Verification items for the finished model (mm, model axes). A direction names the side the tool comes from. Coordinates: 2 decimals unless noted, no trailing zeros. Order: outer loops, then holes, each group sorted by start corner. A loop starts at its lowest first (then second) coordinate and runs counter-clockwise, first axis right, second up.
Q1. Cross-section at C-C, the plane z = 8.5. Record the boundary of the cut face in (x, y).
Q2. Cross-section at D-D, the plane z = 2.5. Record the boundary of the cut face in (x, y).
Q3. Thickness scan on line 1 (Y direction, x = 20.5, z = 5.5); line 2 (Y direction, x = -38.5, z = 4.25); line 3 (X direction, y = -21, z = 4.5). Record the ranges inside material, lowest first.
Q4. Set-up check for faces 1 (the flat face through (15.98, 33.95, 2.53)), 2 (the flat face through (-28, 16, 10)), 3 (the cylindrical face through (16.71, 32.91, 8.5)): record each of +Z, -Z, +X, -X, +Y, -Y from which the full face is reachable in a straight line by a thin tool's end or side.
Q5. Depth check by flat-ended pin: P1, Ø3, axis at x = -38.5, z = 7, coming from the +Y side; P2, Ø1, axis at x = 11.5, z = 6.5, coming from the +Y side; P3, Ø3, axis at y = -21, z = 8, coming from the -X side. Enter the tip coordinate at first touch or a pass-through.
from build123d import *

# Parameters (mm, degrees)
F1_DEPTH = 10
F2_R     = 5
F3_SIZE  = 4.99999


# Not quite as in the source:
# - a fillet or chamfer is up to 0.001 mm smaller than in the source, because OpenCascade refuses the exact size


with BuildPart() as f1:
    # F0 (on Top) → F1 (new body)
    with BuildSketch(Plane.XY):
        Polygon((42.2499991953, 60.7764059144), (-57.7500008047, 60.7764059144), (-57.7500008047, -53.026408835), (-33.2429584743, -53.026408835), (-5.9190154745, 31.4806343348), (42.2499991953, 31.4806343348), align=None)
    extrude(amount=F1_DEPTH)

    # F2
    f2_edges = [f1.edges().sort_by_distance(p)[0] for p in [
        (-57.750001, 3.874999, 10),
        (-19.580987, -10.772887, 10),
        (-45.49648, -53.026409, 10),
        (18.165492, 31.480634, 10),
        (-7.750001, 60.776406, 10),
        (42.249999, 46.12852, 10),
    ]]
    fillet(f2_edges, radius=F2_R)

    # F3 (size 5 in the source; OpenCascade refuses exactly that, so slightly less here)
    f3_edges = [f1.edges().sort_by_distance(p)[0] for p in [
        (18.165492, 31.480634, 0),
        (42.249999, 46.12852, 0),
        (-7.750001, 60.776406, 0),
        (-57.750001, 3.874999, 0),
        (-45.49648, -53.026409, 0),
        (-19.580987, -10.772887, 0),
    ]]
    chamfer(f3_edges, length=F3_SIZE)


solid = f1.part
Check values:
1. outline: (-56.32, -51.6) - (-34.28, -51.6) - (-6.96, 32.91) - (40.82, 32.91) - (40.82, 59.35) - (-56.32, 59.35) - close
2. outline: (-55.25, -50.53) - (-35.06, -50.53) - (-7.74, 33.98) - (39.75, 33.98) - (39.75, 58.28) - (-55.25, 58.28) - close
3. line 1: y = 31.51 to 60.75
3. line 2: y = -52.28 to 60.03
3. line 3: x = -57.25 to -23.41
4. face 1: -Z, +X, -Y
4. face 2: +Z, +X, -X, +Y, -Y
4. face 3: +Z, +X, -Y
5. P1: stops at y = 60.75
5. P2: stops at y = 60.68
5. P3: stops at x = -57.52
